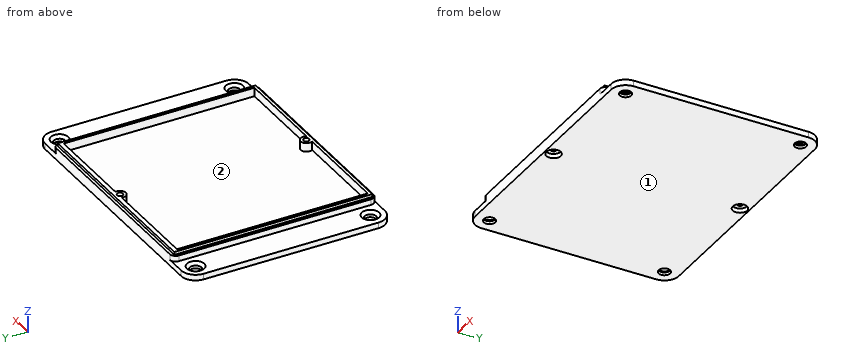
from build123d import *

# Parameters (mm, degrees)
CYLINDER004_R            = 2
CYLINDER004_DEPTH        = 10
ARRAY005_Y_COUNT         = 2
ARRAY005_Y_PITCH         = 60.5
BOX007_W                 = 10
BOX007_H                 = 70.5
BOX007_DEPTH             = 2
ARRAY006_X_COUNT         = 2
ARRAY006_X_PITCH         = 84
CYLINDER003_R            = 2.5
CYLINDER003_DEPTH        = 1.5
ARRAY004_Y_COUNT         = 2
ARRAY004_Y_PITCH         = 64.5
CYLINDER002_R            = 1
CYLINDER002_DEPTH        = 20
ARRAY003_Y_COUNT         = 2
ARRAY003_Y_PITCH         = 64.5
PCB_BOUNDING_BOX_1_W     = 70
PCB_BOUNDING_BOX_1_H     = 66
PCB_BOUNDING_BOX_1_DEPTH = 20
BOX001_W                 = 72
BOX001_H                 = 68.5
BOX001_DEPTH             = 1
BOX_W                    = 74
BOX_H                    = 70.5
BOX_DEPTH                = 4
CYLINDER_R               = 2
CYLINDER_DEPTH           = 3
ARRAY_Y_COUNT            = 2
ARRAY_Y_PITCH            = 64.5
FILLET001_R              = 2
FILLET002_R              = 5
CHAMFER_SIZE             = 1


with BuildPart() as array005:
    # Cylinder004 → Cylinder004 (new body)
    with BuildSketch(Plane(origin=(144.146, -130.588, -4), x_dir=(1, 0, 0), z_dir=(0, 0, 1))):
        Circle(CYLINDER004_R)
    extrude(amount=CYLINDER004_DEPTH)

    # Array005 Y: Array005 ×2


with BuildPart() as array005_1:
    add(array005.part)
    with Locations(*[(0, i * ARRAY005_Y_PITCH, 0) for i in range(1, ARRAY005_Y_COUNT)]):
        add(array005.part)


with BuildPart() as array006:
    # Box007 → Box007 (new body)
    with BuildSketch(Plane(origin=(139.146, -135.588, -4), x_dir=(1, 0, 0), z_dir=(0, 0, 1))):
        with Locations((5, 35.25)):
            Rectangle(BOX007_W, BOX007_H)
    extrude(amount=BOX007_DEPTH)

    # Cut009: cut Array005
    add(array005_1.part, mode=Mode.SUBTRACT)

    # Array006 X: Array006 ×2


with BuildPart() as array006_1:
    add(array006.part)
    with Locations(*[(i * ARRAY006_X_PITCH, 0, 0) for i in range(1, ARRAY006_X_COUNT)]):
        add(array006.part)


with BuildPart() as array004:
    # Cylinder003 → Cylinder003 (new body)
    with BuildSketch(Plane(origin=(187.246, -132.588, -4), x_dir=(1, 0, 0), z_dir=(0, 0, 1))):
        Circle(CYLINDER003_R)
    extrude(amount=CYLINDER003_DEPTH)

    # Array004 Y: Array004 ×2


with BuildPart() as array004_1:
    add(array004.part)
    with Locations(*[(0, i * ARRAY004_Y_PITCH, 0) for i in range(1, ARRAY004_Y_COUNT)]):
        add(array004.part)


with BuildPart() as lochboden:
    # Cylinder002 → Cylinder002 (new body)
    with BuildSketch(Plane(origin=(187.246, -132.588, -4), x_dir=(1, 0, 0), z_dir=(0, 0, 1))):
        Circle(CYLINDER002_R)
    extrude(amount=CYLINDER002_DEPTH)

    # Array003 Y: LochBoden ×2


with BuildPart() as lochboden_1:
    add(lochboden.part)
    with Locations(*[(0, i * ARRAY003_Y_PITCH, 0) for i in range(1, ARRAY003_Y_COUNT)]):
        add(lochboden.part)


with BuildPart() as obj1:
    # PCB_Bounding_Box_1 → PCB_Bounding_Box_1 (new body)
    with BuildSketch(Plane(origin=(151.146, -133.588, -2), x_dir=(1, 0, 0), z_dir=(0, 0, 1))):
        with Locations((35, 33)):
            Rectangle(PCB_BOUNDING_BOX_1_W, PCB_BOUNDING_BOX_1_H)
    extrude(amount=PCB_BOUNDING_BOX_1_DEPTH)


with BuildPart() as obj2:
    # Box001 → Box001 (new body)
    with BuildSketch(Plane(origin=(150.146, -134.588, 0), x_dir=(1, 0, 0), z_dir=(0, 0, 1))):
        with Locations((36, 34.25)):
            Rectangle(BOX001_W, BOX001_H)
    extrude(amount=BOX001_DEPTH)


with BuildPart() as cut:
    # Box → Box (new body)
    with BuildSketch(Plane(origin=(149.146, -135.588, -4), x_dir=(1, 0, 0), z_dir=(0, 0, 1))):
        with Locations((37, 35.25)):
            Rectangle(BOX_W, BOX_H)
    extrude(amount=BOX_DEPTH)

    # Fusion: union obj2
    add(obj2.part)

    # Cut: cut obj1
    add(obj1.part, mode=Mode.SUBTRACT)


with BuildPart() as chamfer_body:
    # Cylinder → Cylinder (new body)
    with BuildSketch(Plane(origin=(187.246, -132.588, -2), x_dir=(1, 0, 0), z_dir=(0, 0, 1))):
        Circle(CYLINDER_R)
    extrude(amount=CYLINDER_DEPTH)

    # Array Y: Chamfer body ×2


with BuildPart() as chamfer_body_1:
    add(chamfer_body.part)
    with Locations(*[(0, i * ARRAY_Y_PITCH, 0) for i in range(1, ARRAY_Y_COUNT)]):
        add(chamfer_body.part)

    # Fusion003: union Cut
    add(cut.part)

    # Cut006: cut LochBoden
    add(lochboden_1.part, mode=Mode.SUBTRACT)

    # Cut008: cut Array004
    add(array004_1.part, mode=Mode.SUBTRACT)

    # Fusion005: union Array006
    add(array006_1.part)

    # Fillet001
    fillet001_edges = [chamfer_body_1.edges().sort_by_distance(p)[0] for p in [
        (149.146, -135.588, -1),
        (149.146, -65.088, -1),
        (223.146, -65.088, -1),
        (223.146, -135.588, -1),
    ]]
    fillet(fillet001_edges, radius=FILLET001_R)

    # Fillet002
    fillet002_edges = [chamfer_body_1.edges().sort_by_distance(p)[0] for p in [
        (139.146, -135.588, -3),
        (233.146, -135.588, -3),
        (139.146, -65.088, -3),
        (233.146, -65.088, -3),
    ]]
    fillet(fillet002_edges, radius=FILLET002_R)

    # Chamfer
    chamfer_edges = [chamfer_body_1.edges().sort_by_distance(p)[0] for p in [
        (142.146, -70.088, -2),
        (142.146, -130.588, -2),
        (226.146, -70.088, -2),
        (226.146, -130.588, -2),
    ]]
    chamfer(chamfer_edges, length=CHAMFER_SIZE)


solid = chamfer_body_1.part
The model under review builds one solid part; all positions refer to its coordinate system, in mm. Face numbers are marked on the shaded views. Round coordinates to 2 decimals unless told otherwise and drop trailing zeros. Loops run counter-clockwise (first coordinate to the right, second up) from the corner with the lowest first, then second, coordinate; pieces in that order, holes last. Notation, with made-up numbers: M 60,48.25 L 67,48.25 A15 ccw 67,73.25 Z; hole C -22,66.5 d5. An arc over 180 degrees is marked long. Answer as a JSON object with one key per item and string values.
Item 1: The part is to be moulded in two halves that separate along Y. For the marked faces 1 and 2, say which applies: +Y half, -Y half, draft (parallel to the pull), parting line (faces both ways), or undercut.
Check sheet entries:
{"face 1": "draft", "face 2": "undercut"}
Item 2: We need section A-A, the plane x = 209.5. State the section outline as (y, z) points, and give its area (4 significant figures).
Check sheet entries:
{"outline": "M -135.59,-4 L -65.09,-4 L -65.09,0 L -66.09,0 L -66.09,1 L -67.59,1 L -67.59,-2 L -133.59,-2 L -133.59,1 L -134.59,1 L -134.59,0 L -135.59,0 Z", "area": "152.5 mm2"}
Item 3: Clearance check with flat-ended pins moving along their axes: P1, Ø5, axis at x = 144.146, y = -130.588, coming from the +Z side; P2, Ø13, axis at x = 228, y = -89.5, coming from the +Z side; P3, Ø5, axis at x = 161, y = -80, coming from the +Z side; P4, Ø0.6, axis at y = -111.5, z = -1, coming from the +X side. State where each tip first meets the part, or that it passes through.
Check sheet entries:
{"P1": "z = -2.5", "P2": "z = 1", "P3": "z = -2", "P4": "x = 223.15"}
Item 4: For line 1 along Y through (x, z) = (177.5, -0.6); line 2 along Y through (x, z) = (157.5, 0.7); line 3 along Y through (x, z) = (228, -3.3), list the stretches that pass through material, from the lowest coordinate up.
Check sheet entries:
{"line 1": "-135.59 to -133.59, -67.59 to -65.09", "line 2": "-134.59 to -133.59, -67.59 to -66.09", "line 3": "-135.59 to -132.58, -128.59 to -72.08, -68.09 to -65.09"}
Item 5: We need section B-B, the plane y = -76. State the section outline as (x, z) points.
Check sheet entries:
{"outline": "M 139.15,-4 L 233.15,-4 L 233.15,-2 L 223.15,-2 L 223.15,0 L 222.15,0 L 222.15,1 L 221.15,1 L 221.15,-2 L 151.15,-2 L 151.15,1 L 150.15,1 L 150.15,0 L 149.15,0 L 149.15,-2 L 139.15,-2 Z"}
